Here's the drawing with two shaded views (mm, measured from the low corner). I have some questions. A direction names the side the tool comes from. Coordinates: 2 decimals unless noted, no trailing zeros. Loops run counter-clockwise (first coordinate to the right, second up) from the corner with the lowest first, then second, coordinate; pieces in that order, holes last. Notation, with made-up numbers: M 43.25,20.25 L 61.25,20.25 A18 ccw 61.25,38.25 Z; hole C -29.5,66.25 d3. An arc over 180 degrees is marked long. Return JSON: item names as keys, results as strings. Group by question number.
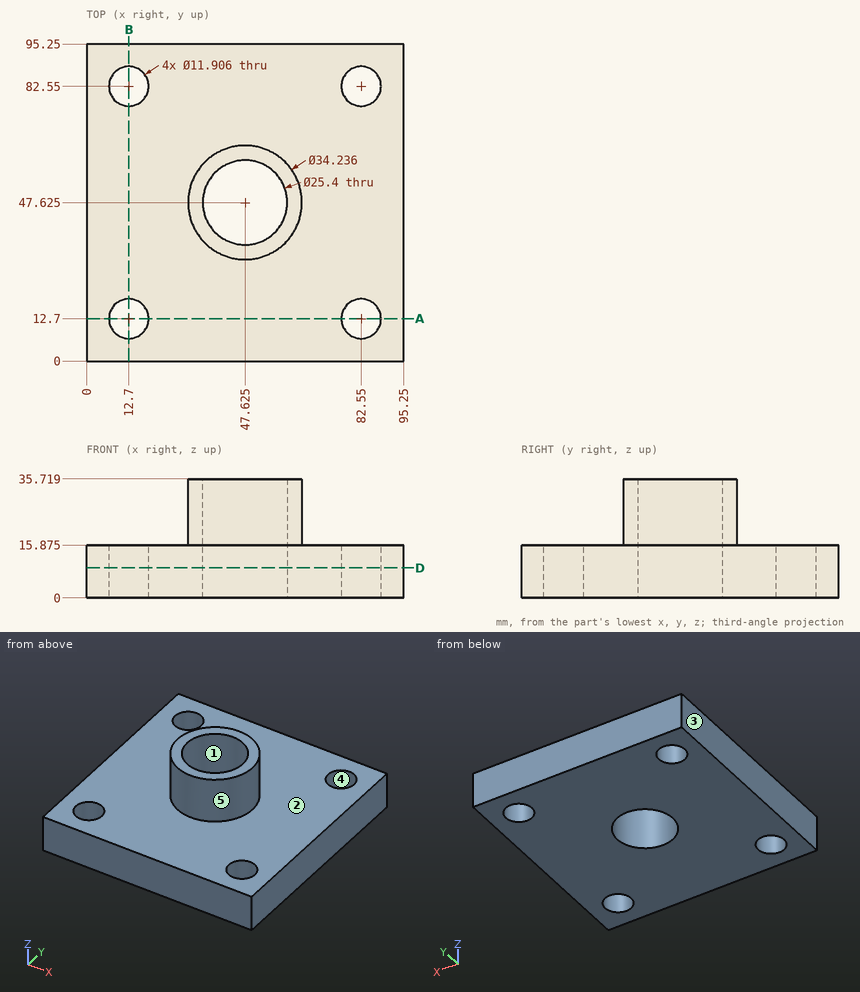
(1) If I drill on L1, parallel to X at y = 82, z = 8; L2, parallel to X at y = 82.55, z = 11, over which ranges is the centre line in solid material (lowest first)? Write a range as [from, to].
(2) Will this pin go through, and if not, where does the flat tip stop? P1, Ø13.5, axis at x = 12.7, y = 12.7, coming from the +Z side (3 decimals).
(3) For the marked faces 1 and 2, which set-ups out of +Z, -Z, +X, -X, +Y, -Y let a thin tool reach every point of the face, with its end or its side?
(4) Imagine slicing it at D-D, the plane z = 9. Write out the boundary of the cut face in (x, y) (3 decimals), then the cut area to 3 significant figures.
(5) Imagine slicing it at A-A, the plane y = 12.7. Write out the boundary of the cut face in (x, z) (3 decimals), then the cut area to 3 significant figures.
(6) We'd pull the mould along Y, two halves only. Please class the marked faces 3, 4 and 5: +Y half, -Y half, draft (parallel to the pull), parting line (faces both ways), or undercut.
Checks:
{
 "1": {"L1": "[0, 6.77], [18.63, 76.62], [88.48, 95.25]", "L2": "[0, 6.75], [18.65, 76.6], [88.5, 95.25]"},
 "2": {"P1": "z = 15.875"},
 "3": {"face 1": "+Z, -Z", "face 2": "+Z"},
 "4": {"outline": "M 0,0 L 95.25,0 L 95.25,95.25 L 0,95.25 Z; hole C 12.7,12.7 d11.906; hole C 12.7,82.55 d11.906; hole C 47.625,47.625 d25.4; hole C 82.55,12.7 d11.906; hole C 82.55,82.55 d11.906", "area": "8,120 mm²"},
 "5": {"outline": "M 0,0 L 6.747,0 L 6.747,15.875 L 0,15.875 Z; M 18.653,0 L 76.597,0 L 76.597,15.875 L 18.653,15.875 Z; M 88.503,0 L 95.25,0 L 95.25,15.875 L 88.503,15.875 Z", "area": "1,130 mm²"},
 "6": {"face 3": "draft", "face 4": "undercut", "face 5": "parting line"}
}
